from build123d import *

# Parameters (mm, degrees)
SKETCH1_W           = 155.4
SKETCH1_H           = 80
BOSS_EXTRUDE1_DEPTH = 5
SKETCH2_W           = 155.4
SKETCH2_H           = 5
BOSS_EXTRUDE2_DEPTH = 75
BOSS_EXTRUDE3_DEPTH = 5
CUT_EXTRUDE2_REACH  = 249.334
SKETCH7_R           = 2.1
CUT_EXTRUDE3_REACH  = 245.822


with BuildPart() as part:
    # Sketch1 → Boss-Extrude1 (new body)
    with BuildSketch(Plane(origin=(0, 0, 0), x_dir=(1, 0, 0), z_dir=(0, 1, 0))):
        with Locations((77.7, 40)):
            Rectangle(SKETCH1_W, SKETCH1_H)
    extrude(amount=BOSS_EXTRUDE1_DEPTH)

    # Sketch2 → Boss-Extrude2 (add)
    with BuildSketch(Plane.XZ):
        with Locations((77.7, -2.5)):
            Rectangle(SKETCH2_W, SKETCH2_H)
    extrude(amount=BOSS_EXTRUDE2_DEPTH)

    # Sketch4 → Boss-Extrude3 (add)
    with BuildSketch(Plane.XY):
        Polygon((131.839983018, -170), (155.4, -75), (0.768966036, -75), (0, -75), (24.328983018, -170), (26.154336071, -170), align=None)
    extrude(amount=-BOSS_EXTRUDE3_DEPTH)

    # Sketch7 → Cut-Extrude2 (cut, up to next)
    with BuildSketch(Plane(origin=(0, 5, 0), x_dir=(1, 0, 0), z_dir=(0, 1, 0)), mode=Mode.PRIVATE) as cut_extrude2_sk1:
        with BuildLine():
            Line((92.7, 20.05), (92.7, 59.95))
            Line((92.7, 59.95), (77.7, 59.95))
            Line((77.7, 59.95), (77.7, 36.45))
            ThreePointArc((77.7, 36.45), (82.331549417, 34.531549417), (84.25, 29.9))
            ThreePointArc((84.25, 29.9), (82.331549417, 25.268450583), (77.7, 23.35))
            Line((77.7, 23.35), (77.7, 20.05))
            Line((77.7, 20.05), (92.7, 20.05))
        make_face()
    cut_extrude2_tool1 = extrude(cut_extrude2_sk1.sketch, amount=-CUT_EXTRUDE2_REACH, mode=Mode.PRIVATE) & part.part
    # Sketch7 → Cut-Extrude2 (cut, up to next)
    with BuildSketch(Plane(origin=(0, 5, 0), x_dir=(1, 0, 0), z_dir=(0, 1, 0)), mode=Mode.PRIVATE) as cut_extrude2_sk2:
        with BuildLine():
            Line((77.7, 36.45), (77.7, 59.95))
            Line((77.7, 59.95), (62.7, 59.95))
            Line((62.7, 59.95), (62.7, 20.05))
            Line((62.7, 20.05), (77.7, 20.05))
            Line((77.7, 20.05), (77.7, 23.35))
            ThreePointArc((77.7, 23.35), (71.15, 29.9), (77.7, 36.45))
        make_face()
    cut_extrude2_tool2 = extrude(cut_extrude2_sk2.sketch, amount=-CUT_EXTRUDE2_REACH, mode=Mode.PRIVATE) & part.part
    # Sketch7 → Cut-Extrude2 (cut, up to next)
    with BuildSketch(Plane(origin=(0, 5, 0), x_dir=(1, 0, 0), z_dir=(0, 1, 0)), mode=Mode.PRIVATE) as cut_extrude2_sk3:
        with BuildLine():
            ThreePointArc((84.25, 29.9), (82.331549417, 34.531549417), (77.7, 36.45))
            Line((77.7, 36.45), (77.7, 23.35))
            ThreePointArc((77.7, 23.35), (82.331549417, 25.268450583), (84.25, 29.9))
        make_face()
    cut_extrude2_tool3 = extrude(cut_extrude2_sk3.sketch, amount=-CUT_EXTRUDE2_REACH, mode=Mode.PRIVATE) & part.part
    # Sketch7 → Cut-Extrude2 (cut, up to next)
    with BuildSketch(Plane(origin=(0, 5, 0), x_dir=(1, 0, 0), z_dir=(0, 1, 0)), mode=Mode.PRIVATE) as cut_extrude2_sk4:
        with BuildLine():
            Line((77.7, 23.35), (77.7, 36.45))
            ThreePointArc((77.7, 36.45), (71.15, 29.9), (77.7, 23.35))
        make_face()
    cut_extrude2_tool4 = extrude(cut_extrude2_sk4.sketch, amount=-CUT_EXTRUDE2_REACH, mode=Mode.PRIVATE) & part.part
    # Sketch7 → Cut-Extrude2 (cut, up to next)
    with BuildSketch(Plane(origin=(0, 5, 0), x_dir=(1, 0, 0), z_dir=(0, 1, 0)), mode=Mode.PRIVATE) as cut_extrude2_sk5:
        with BuildLine():
            ThreePointArc((84.25, 29.9), (82.331549417, 34.531549417), (77.7, 36.45))
            Line((77.7, 36.45), (77.7, 23.35))
            ThreePointArc((77.7, 23.35), (82.331549417, 25.268450583), (84.25, 29.9))
        make_face()
    cut_extrude2_tool5 = extrude(cut_extrude2_sk5.sketch, amount=-CUT_EXTRUDE2_REACH, mode=Mode.PRIVATE) & part.part
    # Sketch7 → Cut-Extrude2 (cut, up to next)
    with BuildSketch(Plane(origin=(0, 5, 0), x_dir=(1, 0, 0), z_dir=(0, 1, 0)), mode=Mode.PRIVATE) as cut_extrude2_sk6:
        with BuildLine():
            Line((77.7, 23.35), (77.7, 36.45))
            ThreePointArc((77.7, 36.45), (71.15, 29.9), (77.7, 23.35))
        make_face()
    cut_extrude2_tool6 = extrude(cut_extrude2_sk6.sketch, amount=-CUT_EXTRUDE2_REACH, mode=Mode.PRIVATE) & part.part
    # Sketch7 → Cut-Extrude2 (cut, up to next)
    with BuildSketch(Plane(origin=(0, 5, 0), x_dir=(1, 0, 0), z_dir=(0, 1, 0)), mode=Mode.PRIVATE) as cut_extrude2_sk7:
        with Locations(Location((82.625, 15.288854382, 0), (0, 0, 270))):
            Circle(SKETCH7_R)
    cut_extrude2_tool7 = extrude(cut_extrude2_sk7.sketch, amount=-CUT_EXTRUDE2_REACH, mode=Mode.PRIVATE) & part.part
    # Sketch7 → Cut-Extrude2 (cut, up to next)
    with BuildSketch(Plane(origin=(0, 5, 0), x_dir=(1, 0, 0), z_dir=(0, 1, 0)), mode=Mode.PRIVATE) as cut_extrude2_sk8:
        with Locations(Location((72.775, 15.288854382, 0), (0, 0, 270))):
            Circle(SKETCH7_R)
    cut_extrude2_tool8 = extrude(cut_extrude2_sk8.sketch, amount=-CUT_EXTRUDE2_REACH, mode=Mode.PRIVATE) & part.part
    # Sketch7 → Cut-Extrude2 (cut, up to next)
    with BuildSketch(Plane(origin=(0, 5, 0), x_dir=(1, 0, 0), z_dir=(0, 1, 0)), mode=Mode.PRIVATE) as cut_extrude2_sk9:
        with Locations(Location((72.775, 64.711145618, 0), (0, 0, 270))):
            Circle(SKETCH7_R)
    cut_extrude2_tool9 = extrude(cut_extrude2_sk9.sketch, amount=-CUT_EXTRUDE2_REACH, mode=Mode.PRIVATE) & part.part
    # Sketch7 → Cut-Extrude2 (cut, up to next)
    with BuildSketch(Plane(origin=(0, 5, 0), x_dir=(1, 0, 0), z_dir=(0, 1, 0)), mode=Mode.PRIVATE) as cut_extrude2_sk10:
        with Locations(Location((82.625, 64.711145618, 0), (0, 0, 270))):
            Circle(SKETCH7_R)
    cut_extrude2_tool10 = extrude(cut_extrude2_sk10.sketch, amount=-CUT_EXTRUDE2_REACH, mode=Mode.PRIVATE) & part.part
    add(cut_extrude2_tool1.solids().sort_by_distance((85.798921, 5, -41.281564))[0], mode=Mode.SUBTRACT)
    add(cut_extrude2_tool2.solids().sort_by_distance((69.601079, 5, -41.281564))[0], mode=Mode.SUBTRACT)
    add(cut_extrude2_tool3.solids().sort_by_distance((80.479906, 5, -29.9))[0], mode=Mode.SUBTRACT)
    add(cut_extrude2_tool4.solids().sort_by_distance((74.920094, 5, -29.9))[0], mode=Mode.SUBTRACT)
    add(cut_extrude2_tool5.solids().sort_by_distance((80.479906, 5, -29.9))[0], mode=Mode.SUBTRACT)
    add(cut_extrude2_tool6.solids().sort_by_distance((74.920094, 5, -29.9))[0], mode=Mode.SUBTRACT)
    add(cut_extrude2_tool7.solids().sort_by_distance((82.625, 5, -15.288854))[0], mode=Mode.SUBTRACT)
    add(cut_extrude2_tool8.solids().sort_by_distance((72.775, 5, -15.288854))[0], mode=Mode.SUBTRACT)
    add(cut_extrude2_tool9.solids().sort_by_distance((72.775, 5, -64.711146))[0], mode=Mode.SUBTRACT)
    add(cut_extrude2_tool10.solids().sort_by_distance((82.625, 5, -64.711146))[0], mode=Mode.SUBTRACT)

    # Sketch8 → Cut-Extrude3 (cut, up to next)
    with BuildSketch(Plane.XY, mode=Mode.PRIVATE) as cut_extrude3_sk1:
        Polygon((25, -71.849651243), (25, -15), (15, -15), (15, -73.109790746), (34.69116416, -150), (45.013879029, -150), align=None)
    cut_extrude3_tool1 = extrude(cut_extrude3_sk1.sketch, amount=-CUT_EXTRUDE3_REACH, mode=Mode.PRIVATE) & part.part
    # Sketch8 → Cut-Extrude3 (cut, up to next)
    with BuildSketch(Plane.XY, mode=Mode.PRIVATE) as cut_extrude3_sk2:
        Polygon((45, -15), (35, -15), (35, -70.589511741), (55.336593898, -150), (65.659308767, -150), (45, -69.329372238), align=None)
    cut_extrude3_tool2 = extrude(cut_extrude3_sk2.sketch, amount=-CUT_EXTRUDE3_REACH, mode=Mode.PRIVATE) & part.part
    # Sketch8 → Cut-Extrude3 (cut, up to next)
    with BuildSketch(Plane.XY, mode=Mode.PRIVATE) as cut_extrude3_sk3:
        Polygon((90.421655908, -149.945595989), (100.744271122, -149.900237253), (120.731733413, -70.401155194), (120.487469184, -14.812180114), (110.487565723, -14.856120818), (110.726292811, -69.184968561), align=None)
    cut_extrude3_tool3 = extrude(cut_extrude3_sk3.sketch, amount=-CUT_EXTRUDE3_REACH, mode=Mode.PRIVATE) & part.part
    # Sketch8 → Cut-Extrude3 (cut, up to next)
    with BuildSketch(Plane.XY, mode=Mode.PRIVATE) as cut_extrude3_sk4:
        Polygon((111.066886336, -149.854878517), (121.389501549, -149.809519781), (140.742614617, -72.833528461), (140.487276104, -14.724298705), (130.487372644, -14.768239409), (130.737174015, -71.617341828), align=None)
    cut_extrude3_tool4 = extrude(cut_extrude3_sk4.sketch, amount=-CUT_EXTRUDE3_REACH, mode=Mode.PRIVATE) & part.part
    add(cut_extrude3_tool1.solids().sort_by_distance((25.777168, -83.022875, 0))[0], mode=Mode.SUBTRACT)
    add(cut_extrude3_tool2.solids().sort_by_distance((46.155254, -83.015898, 0))[0], mode=Mode.SUBTRACT)
    add(cut_extrude3_tool3.solids().sort_by_distance((109.631189, -82.876438, 0))[0], mode=Mode.SUBTRACT)
    add(cut_extrude3_tool4.solids().sort_by_distance((130.00911, -82.793873, 0))[0], mode=Mode.SUBTRACT)


solid = part.part
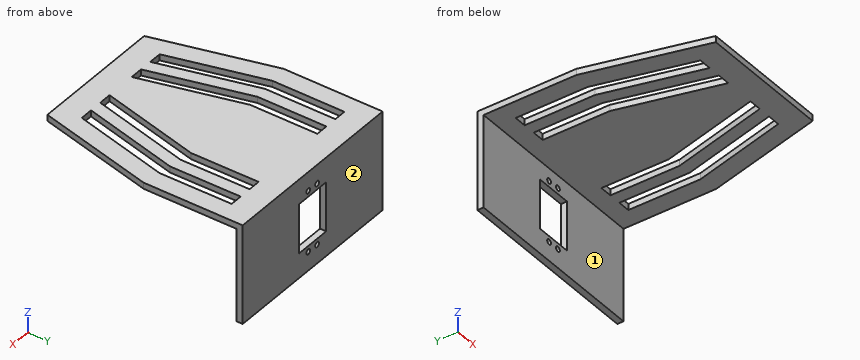
Input: part model. Units: mm. Frame: model coordinates. Face numbers are marked on the shaded views. A direction names the side the tool comes from. Coordinates: 2 decimals unless noted, no trailing zeros. Order: outer loops, then holes, each group sorted by start corner. A loop starts at its lowest first (then second) coordinate and runs counter-clockwise, first axis right, second up. Notation, with made-up numbers: M 79.25,6.25 L 122.25,6.25 A11 cw 122.25,23.25 Z; hole C -30,4.25 d7. An arc over 180 degrees is marked long. Answer in a Markdown table with one row per item.
(1) Section query A-A, the plane z = -31.5. Output: boundary loops of the cut face in (x, y).
Numbers:
| item | result |
|---|---|
| outline | M 0,0 L 62.7,0 L 62.7,5 L 0,5 Z; M 92.7,0 L 155.4,0 L 155.4,5 L 92.7,5 Z |
(2) Access query for the marked faces 1 and 2. Directions: +Z, -Z, +X, -X, +Y, -Y. A direction counts if a zero-diameter tool reaches every point of the face in a straight line with its end or side. Return the directions, or none.
Numbers:
| item | result |
|---|---|
| face 1 | -Z, +X, -X, -Y |
| face 2 | +Z, -Z, +X, -X, +Y |
(3) Section query B-B, the plane y = -83.5. Output: boundary loops of the cut face in (x, z).
Numbers:
| item | result |
|---|---|
| outline | M 2.18,-5 L 17.66,-5 L 17.66,0 L 2.18,0 Z; M 27.98,-5 L 38.31,-5 L 38.31,0 L 27.98,0 Z; M 48.63,-5 L 107.13,-5 L 107.13,0 L 48.63,0 Z; M 117.44,-5 L 127.75,-5 L 127.75,0 L 117.44,0 Z; M 138.06,-5 L 153.29,-5 L 153.29,0 L 138.06,0 Z |
(4) Section query C-C, the plane x = 108. Output: boundary loops of the cut face in (y, z).
Numbers:
| item | result |
|---|---|
| outline | M -170,-5 L -121.04,-5 L -121.04,0 L -170,0 Z; M -80.03,-5 L 0,-5 L 0,-80 L 5,-80 L 5,0 L -80.03,0 Z |
(5) Contact query for a flat-ended pin moving along its axis: pin 1 Ø2 at (x, z) = (65.5, -68.5) entering from -Y. Output: stop coordinate, or through.
Numbers:
| item | result |
|---|---|
| pin 1 | stops at y = 0 |
(6) Material intervals for line 1 (Z direction, x = 98, y = -112.5); line 2 (Y direction, x = 125, z = -54.5), sorted ascending. Write a range as [from, to].
Numbers:
| item | result |
|---|---|
| line 1 | z = [-5, 0] |
| line 2 | y = [0, 5] |
(7) Section query D-D, the plane y = -45. Output: boundary loops of the cut face in (x, z).
Numbers:
| item | result |
|---|---|
| outline | M 0,-5 L 15,-5 L 15,0 L 0,0 Z; M 25,-5 L 35,-5 L 35,0 L 25,0 Z; M 45,-5 L 110.62,-5 L 110.62,0 L 45,0 Z; M 120.62,-5 L 130.62,-5 L 130.62,0 L 120.62,0 Z; M 140.62,-5 L 155.4,-5 L 155.4,0 L 140.62,0 Z |
